```python
from build123d import *

# Parameters (mm, degrees)
SKETCH1_R           = 1.6
BOSS_EXTRUDE1_DEPTH = 4
CHAMFER1_SIZE       = 1


with BuildPart() as part:
    # Sketch1 → Boss-Extrude1 (new body)
    with BuildSketch(Plane(origin=(0, 0, 0), x_dir=(0, 0, -1), z_dir=(1, 0, 0))):
        with BuildLine():
            Line((14, 0), (25, 0))
            ThreePointArc((25, 0), (0, 25), (-25, 0))
            Line((-25, 0), (-14, 0))
            ThreePointArc((-14, 0), (0, 14), (14, 0))
        make_face()
        with Locations((14, 14.282856857)):
            Circle(SKETCH1_R, mode=Mode.SUBTRACT)
        with Locations((-14, 14.282856857)):
            Circle(SKETCH1_R, mode=Mode.SUBTRACT)
    extrude(amount=BOSS_EXTRUDE1_DEPTH)

    # Chamfer1
    chamfer1_edges = [part.edges().sort_by_distance(p)[0] for p in [
        (4, 25, 0),
        (4, 14, 0),
    ]]
    chamfer(chamfer1_edges, length=CHAMFER1_SIZE)


solid = part.part
```
Geometry: final body of the model. Coordinates: model frame, mm. Round coordinates to 2 decimals unless told otherwise and drop trailing zeros. Loops run counter-clockwise (first coordinate to the right, second up) from the corner with the lowest first, then second, coordinate; pieces in that order, holes last. Notation, with made-up numbers: (-40, 75.25) -> (-5, 75.25) arc R36 cw to (-5, 112.25) -> close; hole circle Ø2 at (64.25, -5.75). An arc over 180 degrees is marked (long way). Use one line per item in the form item = value. Start each with the question number.
1) Section A-A on x = 2.1. Output: boundary loops of the cut face in (y, z).
2) Section B-B on z = 0. Output: boundary loops of the cut face in (x, y), then the cut area to 3 significant figures.
3) Line query: L1, parallel to Z at x = 1.7, y = 15.5; L2, parallel to Z at x = 2.9, y = 14.5; L3, parallel to Z at x = 1.95, y = 2.75. Output: solid intervals per line, ascending.
4) Draft query along Z for faces 1 (the flat face through (4, 18, 0)), 2 (the cylindrical face through (1.479, 24.994, -0.55)), 3 (the cylindrical face through (1.972, 15.364, 15.179)). Return one class per face: released by +Z, released by -Z, zero draft, split by the parting line, or undercut.
5) First-contact query: P1, Ø3, axis at y = 14.28, z = 14, coming from the -X side. Flat tip, straight axial feed; report the tip coordinate or a pass-through.
Response:
q1.outline = (0, -25) arc R25 ccw to (0, 25) -> (0, 14) arc R14 cw to (0, -14) -> close; hole circle Ø3.2 at (14.28, -14); hole circle Ø3.2 at (14.28, 14)
q2.outline = (0, 14) -> (3, 14) -> (4, 15) -> (4, 24) -> (3, 25) -> (0, 25) -> close
q2.area = 43.0 mm^2
q3.L1 = -19.62 to -15.04, -12.96 to 12.96, 15.04 to 19.62
q3.L2 = -20.37 to -15.59, -12.41 to 12.41, 15.59 to 20.37
q3.L3 = -24.85 to -13.73, 13.73 to 24.85
q4.face_1 = zero draft
q4.face_2 = split by the parting line
q4.face_3 = undercut
q5.P1 = through
